The model under review builds one solid part; all positions refer to its coordinate system, in mm. A direction names the side the tool comes from. Round coordinates to 2 decimals unless told otherwise and drop trailing zeros. Loops run counter-clockwise (first coordinate to the right, second up) from the corner with the lowest first, then second, coordinate; pieces in that order, holes last. Notation, with made-up numbers: (-26.5, 78) -> (0.5, 78) arc R14 cw to (0.5, 97) -> close; hole circle Ø3 at (21.5, -22). An arc over 180 degrees is marked (long way). Use a Markdown table: item, result. Add a question column.
1) Consider section B-B on z = 29. Give the boundary of the cut face in (x, y).
2) Consider section A-A on y = 12.5. Give the boundary of the cut face in (x, z).
3) Mouldability with a two-part tool opening along X and no side actions: class faces 1 (the cylindrical face through (11.286, 3.944, 30.494)), 2 (the flat face through (13, 23, 4)), 3 (the cylindrical face through (1.06, 36.21, 1.97)) as released by +X, released by -X, zero draft, split by the parting line, or undercut.
4) Consider section D-D on y = 33. Give the boundary of the cut face in (x, z).
5) Wall thickness on probe 1 along Z at (x, y) = (16.5, 38); probe 2 along Y at (x, z) = (11, 0.95); probe 3 along Y at (x, z) = (17.5, 38): over which ranges is each line inside the solid? List them lowest first.
6) Consider section C-C on x = 11. Give the boundary of the cut face in (y, z), plus the area to 3 significant figures.
7) For faces 4 (the cylindrical face through (22.176, 21.2, 45.528)), 5 (the flat face through (13, 23, 43.5)), list the 3-axis set-ups (+Z, -Z, +X, -X, +Y, -Y) from which the entire face can be reached by the end or side of a thin tool; tool diameter is ignored.
from build123d import *

# Parameters (mm, degrees)
BOSS_EXTRUDE1_DEPTH = 4
SKETCH2_W           = 22
SKETCH2_H           = 8
BOSS_EXTRUDE2_DEPTH = 39.5
BOSS_EXTRUDE3_DEPTH = 4
FILLET1_R           = 3
SKETCH4_R           = 6.5
CUT_EXTRUDE1_DEPTH  = 72.375766196
CUT_EXTRUDE2_REACH  = 73.376
SKETCH5_R           = 6.5


with BuildPart() as part:
    # Sketch1 → Boss-Extrude1 (new body)
    with BuildSketch(Plane.XY):
        with BuildLine():
            Line((0, 0), (22, 0))
            Line((22, 0), (22, 21.301960973))
            ThreePointArc((22, 21.301960973), (22.819670179, 40.735550707), (3.764629611, 44.63961245))
            ThreePointArc((3.764629611, 44.63961245), (4.991727504, 42.319183704), (3.923405192, 39.92150853))
            ThreePointArc((3.923405192, 39.92150853), (1.028978415, 36.145291009), (0, 31.5))
            Line((0, 31.5), (0, 0))
        make_face()
    extrude(amount=BOSS_EXTRUDE1_DEPTH)

    # Sketch2 → Boss-Extrude2 (add)
    with BuildSketch(Plane.XY.offset(4)):
        with Locations((11, 4)):
            Rectangle(SKETCH2_W, SKETCH2_H)
    extrude(amount=BOSS_EXTRUDE2_DEPTH)

    # Sketch3 → Boss-Extrude3 (add)
    with BuildSketch(Plane.XY.offset(43.5)):
        with BuildLine():
            Line((0, 0), (22, 0))
            Line((22, 0), (22, 21.301960973))
            ThreePointArc((22, 21.301960973), (22.822920693, 40.731389185), (3.773882637, 44.644703414))
            ThreePointArc((3.773882637, 44.644703414), (4.999346476, 42.323411278), (3.929336293, 39.926488874))
            ThreePointArc((3.929336293, 39.926488874), (1.030614343, 36.148800879), (0, 31.5))
            Line((0, 31.5), (0, 0))
        make_face()
    extrude(amount=BOSS_EXTRUDE3_DEPTH)

    # Fillet1
    fillet1_edges = [part.edges().sort_by_distance(p)[0] for p in [
        (22, 21.301960973, 2),
        (22, 21.301960973, 45.5),
    ]]
    fillet(fillet1_edges, radius=FILLET1_R)

    # Sketch4 → Cut-Extrude1 (cut, through all)
    with BuildSketch(Plane.XY.offset(47.5)):
        with Locations((11, 31.5)):
            Circle(SKETCH4_R)
    extrude(amount=-CUT_EXTRUDE1_DEPTH, mode=Mode.SUBTRACT)

    # Sketch5 → Cut-Extrude2 (cut, up to next)
    with BuildSketch(Plane(origin=(0, 0, 0), x_dir=(-1, 0, 0), z_dir=(0, -1, 0)), mode=Mode.PRIVATE) as cut_extrude2_sk1:
        with Locations(Location((-11, -24, 0), (0, 0, 90))):
            Circle(SKETCH5_R)
    cut_extrude2_tool1 = extrude(cut_extrude2_sk1.sketch, amount=-CUT_EXTRUDE2_REACH, mode=Mode.PRIVATE) & part.part
    add(cut_extrude2_tool1.solids().sort_by_distance((11, 0, 24))[0], mode=Mode.SUBTRACT)


solid = part.part
Result set:
| question | item | result |
|---|---|---|
| 1 | outline | (0, 0) -> (6.85, 0) -> (6.85, 8) -> (0, 8) -> close; (15.15, 0) -> (22, 0) -> (22, 8) -> (15.15, 8) -> close |
| 2 | outline | (0, 0) -> (22, 0) -> (22, 4) -> (0, 4) -> close; (0, 43.5) -> (22, 43.5) -> (22, 47.5) -> (0, 47.5) -> close |
| 3 | face 1 | undercut |
| 3 | face 2 | zero draft |
| 3 | face 3 | released by -X |
| 4 | outline | (0.1, 0) -> (4.68, 0) -> (4.68, 4) -> (0.1, 4) -> close; (0.1, 43.5) -> (4.68, 43.5) -> (4.68, 47.5) -> (0.1, 47.5) -> close; (17.32, 0) -> (25.92, 0) -> (25.92, 4) -> (17.32, 4) -> close; (17.32, 43.5) -> (25.92, 43.5) -> (25.92, 47.5) -> (17.32, 47.5) -> close |
| 5 | probe 1 | 0 to 4, 43.5 to 47.5 |
| 5 | probe 2 | 0 to 25, 38 to 46.5 |
| 5 | probe 3 | 0 to 8 |
| 6 | outline | (0, 0) -> (25, 0) -> (25, 4) -> (8, 4) -> (8, 17.5) -> (0, 17.5) -> close; (0, 30.5) -> (8, 30.5) -> (8, 43.5) -> (25, 43.5) -> (25, 47.5) -> (0, 47.5) -> close; (38, 0) -> (46.5, 0) -> (46.5, 4) -> (38, 4) -> close; (38, 43.5) -> (46.5, 43.5) -> (46.5, 47.5) -> (38, 47.5) -> close |
| 6 | area | 480 mm2 |
| 7 | face 4 | +Z, -Z, +X, -Y |
| 7 | face 5 | +X, -X, +Y |
